Geometry: final body of the model. Coordinates: model frame, mm. A direction names the side the tool comes from. Give positions to 0.01 mm unless a question says otherwise; leave off trailing zeros. Write each loop counter-clockwise with the first axis right and the second up, starting at its lowest first coordinate (ties: lowest second). Pieces come first, ordered by that corner, then holes.
Q1. Pin query (flat end, axial travel): pin 1 (23 mm diameter, centred on x = -6.5, z = -3.5, fed in from -Y) (1 decimal). Return the tip coordinate at first contact, or that it passes through.
Q2. Cut plane D-D on y = -41.5. Return the cut outline in (x, z).
Q3. Cut plane C-C on z = 39.5. Return the cut outline in (x, y).
Q4. Cut plane B-B on x = 0. Return the cut outline in (y, z), plus the area to 3 significant figures.
Q5. Reachability of faces 1 (the face through (-26, 38.1, -1)), 2 (the face through (50.98, -4.38, 10.61)), 3 (the face through (27, 63.5, 1)) from +Z, -Z, +X, -X, +Y, -Y: full face, straight path, thin tool, end or side. Return the list, or none.
Q6. Cut plane A-A on y = 27. Return the cut outline in (x, z), plus the area to 3 significant figures.
Q7. Line query: L1, parallel to X at y = 7.5, z = -10.5; L2, parallel to Z at x = 0, y = 48.25. Output: solid intervals per line, ascending.
Q8. Draft query along X for faces 4 (the face through (5.506, -50.622, -24.796)), 5 (the face through (63.5, -1, -1)), 6 (the face through (-63.5, -1, -1)), 7 (the face through (50.98, 4.51, 10.31)). Return one class per face: pulls with the +X half, pulls with the -X half, needs draft (parallel to the pull), parting line crosses it, or undercut.
```python
from build123d import *

# Parameters (mm, degrees)
F1_W     = 127
F1_H     = 127
F2_DEPTH = 63.5
F3_W     = 76.2
F3_H     = 76.2
F4_DEPTH = 135.636
F6_DEPTH = 146.304
F7_R     = 25.4
F8_DEPTH = 141.986


# Not quite as in the source:
# - a variable given as a bare number and used for a length is read in inches; the dataset says mm whatever the document's units were


with BuildPart() as f2:
    # F1 (on Front) → F2 (new body, symmetric)
    with BuildSketch(Plane.XZ):
        Rectangle(F1_W, F1_H)
    extrude(amount=F2_DEPTH, both=True)

    # F3 (on face) → F4 (cut)
    with BuildSketch(Plane(origin=(0, 0, -63.5), x_dir=(1, 0, 0), z_dir=(0, 0, -1))):
        Rectangle(F3_W, F3_H)
    extrude(amount=-F4_DEPTH, mode=Mode.SUBTRACT)

    # F5 (on face) → F6 (cut)
    with BuildSketch(Plane.YZ.offset(63.5)):
        Polygon((8.8900011033, 0), (0, 20.9176484495), (-8.8900011033, 0), align=None)
    extrude(amount=-F6_DEPTH, mode=Mode.SUBTRACT)

    # F7 (on face) → F8 (cut)
    with BuildSketch(Plane(origin=(0, 63.5, 0), x_dir=(-1, 0, 0), z_dir=(0, 1, 0))):
        Circle(F7_R)
    extrude(amount=-F8_DEPTH, mode=Mode.SUBTRACT)


solid = f2.part
```
Data:
1. pin 1: passes through
2. outline: (-63.5, -63.5) - (63.5, -63.5) - (63.5, 63.5) - (-63.5, 63.5) - close; hole circle Ø50.8 at (0, 0)
3. outline: (-63.5, -63.5) - (63.5, -63.5) - (63.5, 63.5) - (-63.5, 63.5) - close; hole (-38.1, -38.1) - (38.1, -38.1) - (38.1, 38.1) - (-38.1, 38.1) - close
4. outline: (-63.5, -63.5) - (-38.1, -63.5) - (-38.1, -25.4) - (-63.5, -25.4) - close; (-63.5, 25.4) - (-38.1, 25.4) - (-38.1, 63.5) - (-63.5, 63.5) - close; (38.1, -63.5) - (63.5, -63.5) - (63.5, -25.4) - (38.1, -25.4) - close; (38.1, 25.4) - (63.5, 25.4) - (63.5, 63.5) - (38.1, 63.5) - close
4. area: 3,870 mm2
5. face 1: +Z, -Z
5. face 2: +X, -X
5. face 3: +Z, -Z, +X, -X, +Y
6. outline: (-63.5, -63.5) - (-38.1, -63.5) - (-38.1, 63.5) - (-63.5, 63.5) - close; (38.1, -63.5) - (63.5, -63.5) - (63.5, 63.5) - (38.1, 63.5) - close
6. area: 6,450 mm2
7. L1: x = -63.5 to -38.1, 38.1 to 63.5
7. L2: z = -63.5 to -25.4, 25.4 to 63.5
8. face 4: undercut
8. face 5: pulls with the +X half
8. face 6: pulls with the -X half
8. face 7: needs draft
